Design review of the part built by this model. Coordinates are the model's own, in mm. Face numbers are marked on the shaded views. A direction names the side the tool comes from. Round coordinates to 2 decimals unless told otherwise and drop trailing zeros. Write each loop counter-clockwise with the first axis right and the second up, starting at its lowest first coordinate (ties: lowest second). Pieces come first, ordered by that corner, then holes. Notation, with made-up numbers: M -16.75,23.25 L 3.25,23.25 A22 cw 3.25,47.25 Z; hole C 79.5,16 d5. An arc over 180 degrees is marked long. Use CSV: the item, a comma, the result in double quotes.
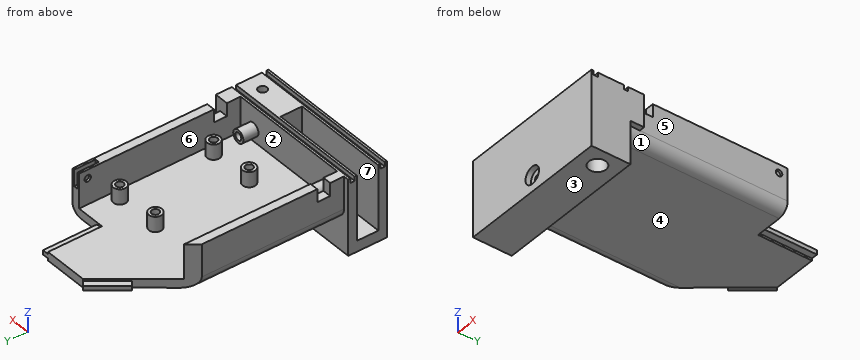
from build123d import *

# Parameters (mm, degrees)
SKETCH1_W                 = 65
SKETCH1_H                 = 40
BOSS_EXTRUDE1_DEPTH       = 100
SHELL1_T                  = -4
FILLET1_R                 = 5
CUT_EXTRUDE1_DEPTH        = 108.033873143
CUT_EXTRUDE1_DEPTH_BACK   = 108.033873143
CUT_EXTRUDE2_DEPTH        = 108.033873143
CUT_EXTRUDE2_DEPTH_BACK   = 108.033873143
SKETCH3_W                 = 17.5
SKETCH3_H                 = 25
SKETCH5_W                 = 2
SKETCH5_H                 = 25
BOSS_EXTRUDE2_DEPTH       = 3
SKETCH6_W                 = 2
SKETCH6_H                 = 18
BOSS_EXTRUDE3_DEPTH       = 3
SKETCH8_W                 = 70
SKETCH8_H                 = 70
BOSS_EXTRUDE4_DEPTH       = 18
SKETCH10_W                = 60
SKETCH10_H                = 10
CUT_EXTRUDE4_DEPTH        = 45
SKETCH23_W                = 2
SKETCH23_H                = 15
CUT_EXTRUDE10_DEPTH       = 10
CUT_EXTRUDE12_DEPTH       = 114.254624289
CUT_EXTRUDE12_DEPTH_BACK  = 114.254624289
SKETCH27_W                = 70
SKETCH27_H                = 35
SKETCH29_W                = 70
SKETCH29_H                = 2
CUT_EXTRUDE13_DEPTH       = 2
SKETCH30_W                = 70
SKETCH30_H                = 2
CUT_EXTRUDE14_DEPTH       = 2
CUT_EXTRUDE15_DEPTH       = 114.254624289
CUT_EXTRUDE15_DEPTH_BACK  = 114.254624289
SKETCH31_R                = 2
SKETCH33_R                = 4
CUT_EXTRUDE16_DEPTH       = 15
CUT_EXTRUDE17_DEPTH       = 114.254624289
CUT_EXTRUDE17_DEPTH_BACK  = 114.254624289
SKETCH34_R                = 1.5
SKETCH35_R                = 4
CUT_EXTRUDE18_DEPTH       = 2.5
SKETCH39_R                = 3
BOSS_EXTRUDE7_DEPTH       = 7
SKETCH40_R                = 1.75
CUT_EXTRUDE20_DEPTH       = 4
LPATTERN4_COUNT           = 2
LPATTERN4_PITCH           = 43.5
CUT_EXTRUDE21_DEPTH       = 128.113570962
CUT_EXTRUDE21_DEPTH_BACK  = 128.113570962
SKETCH41_W                = 6
SKETCH41_H                = 6
SKETCH42_W                = 15
SKETCH42_H                = 6.4
BOSS_EXTRUDE10_DEPTH      = 2.5
CUT_EXTRUDE22_DEPTH       = 128.113570962
CUT_EXTRUDE22_DEPTH_BACK  = 10
SKETCH43_R                = 1.5
SKETCH37_R                = 3
BOSS_EXTRUDE6_DEPTH       = 7
SKETCH38_R                = 1.75
CUT_EXTRUDE19_DEPTH       = 4
LPATTERN1_COUNT           = 2
LPATTERN1_PITCH           = 21
LPATTERN2_COUNT           = 2
LPATTERN2_PITCH           = 43.5
LPATTERN2_COPY_1_SKETCH_R = 3
LPATTERN2_COPY_1_DEPTH    = 7
LPATTERN2_COPY_2_SKETCH_R = 1.75
LPATTERN2_COPY_2_DEPTH    = 4


with BuildPart() as part:
    # Sketch1 → Boss-Extrude1 (new body)
    with BuildSketch(Plane(origin=(0, 0, 0), x_dir=(1, 0, 0), z_dir=(0, 1, 0))):
        Rectangle(SKETCH1_W, SKETCH1_H)
    extrude(amount=BOSS_EXTRUDE1_DEPTH)

    # Shell1
    shell1_openings = [part.faces().sort_by_distance(p)[0] for p in [
        (0, 100, 0),
        (0, 0, 0),
    ]]
    offset(amount=SHELL1_T, openings=shell1_openings, kind=Kind.INTERSECTION)

    # Fillet1
    fillet1_edges = [part.edges().sort_by_distance(p)[0] for p in [
        (32.5, 50, 20),
        (-32.5, 50, 20),
        (-32.5, 50, -20),
        (32.5, 50, -20),
    ]]
    fillet(fillet1_edges, radius=FILLET1_R)

    # Sketch2 → Cut-Extrude1 (cut, two sides: drawn at the far end of the back side and taken through both)
    with BuildSketch(Plane.XY.offset(-CUT_EXTRUDE1_DEPTH_BACK)):
        Polygon((-5.5, 100), (-32.5, 66), (-32.5, 100), align=None)
    extrude(amount=CUT_EXTRUDE1_DEPTH + CUT_EXTRUDE1_DEPTH_BACK, mode=Mode.SUBTRACT)

    # Sketch3 → Cut-Extrude2 (cut, two sides: drawn at the far end of the back side and taken through both)
    with BuildSketch(Plane.XY.offset(-CUT_EXTRUDE2_DEPTH_BACK)):
        with Locations((23.75, 87.5)):
            Rectangle(SKETCH3_W, SKETCH3_H)
    extrude(amount=CUT_EXTRUDE2_DEPTH + CUT_EXTRUDE2_DEPTH_BACK, mode=Mode.SUBTRACT)

    # Sketch5 → Boss-Extrude2 (add)
    with BuildSketch(Plane(origin=(15, 0, 0), x_dir=(0, 0, -1), z_dir=(1, 0, 0))):
        with Locations((-18, 87.5)):
            Rectangle(SKETCH5_W, SKETCH5_H)
    boss_extrude2 = extrude(amount=BOSS_EXTRUDE2_DEPTH)

    # Mirror1: Boss-Extrude2 across plane
    add(boss_extrude2.mirror(Plane.XY))

    # Sketch6 → Boss-Extrude3 (add)
    with BuildSketch(Plane(origin=(-52.073209549, 41.352254642, 0), x_dir=(0, 0, 1), z_dir=(-0.783110847498294, 0.6218821436015861, 0))):
        with Locations((-18, 65.89073296)):
            Rectangle(SKETCH6_W, SKETCH6_H)
    boss_extrude3 = extrude(amount=BOSS_EXTRUDE3_DEPTH)

    # Mirror2: Boss-Extrude3 across plane
    add(boss_extrude3.mirror(Plane.XY))

    # Sketch8 → Boss-Extrude4 (add)
    with BuildSketch(Plane(origin=(0, 0, 0), x_dir=(1, 0, 0), z_dir=(0, 1, 0))):
        Rectangle(SKETCH8_W, SKETCH8_H)
    extrude(amount=-BOSS_EXTRUDE4_DEPTH)

    # Sketch10 → Cut-Extrude4 (cut)
    with BuildSketch(Plane.ZY.offset(35)):
        with Locations((0, -9)):
            Rectangle(SKETCH10_W, SKETCH10_H)
    extrude(amount=-CUT_EXTRUDE4_DEPTH, mode=Mode.SUBTRACT)

    # Sketch23 → Cut-Extrude10 (cut)
    with BuildSketch(Plane(origin=(0, 75, 0), x_dir=(1, 0, 0), z_dir=(0, 1, 0))):
        with Locations((30.5, 0)):
            Rectangle(SKETCH23_W, SKETCH23_H)
    extrude(amount=-CUT_EXTRUDE10_DEPTH, mode=Mode.SUBTRACT)

    # Sketch27 → Cut-Extrude12 (cut, two sides: drawn at the far end of the back side and taken through both)
    with BuildSketch(Plane(origin=(0, 0, 0), x_dir=(1, 0, 0), z_dir=(0, 1, 0)).offset(-CUT_EXTRUDE12_DEPTH_BACK)):
        with Locations((0, -17.5)):
            Rectangle(SKETCH27_W, SKETCH27_H)
    extrude(amount=CUT_EXTRUDE12_DEPTH + CUT_EXTRUDE12_DEPTH_BACK, mode=Mode.SUBTRACT)

    # Sketch29 → Cut-Extrude13 (cut)
    with BuildSketch(Plane.XY):
        with Locations((0, -2)):
            Rectangle(SKETCH29_W, SKETCH29_H)
    extrude(amount=-CUT_EXTRUDE13_DEPTH, mode=Mode.SUBTRACT)

    # Sketch30 → Cut-Extrude14 (cut)
    with BuildSketch(Plane.XY):
        with Locations((0, -16)):
            Rectangle(SKETCH30_W, SKETCH30_H)
    extrude(amount=-CUT_EXTRUDE14_DEPTH, mode=Mode.SUBTRACT)

    # Sketch31 → Cut-Extrude15 (cut, two sides: drawn at the far end of the back side and taken through both)
    with BuildSketch(Plane.XY.offset(-CUT_EXTRUDE15_DEPTH_BACK)):
        with Locations((27, -9)):
            Circle(SKETCH31_R)
    extrude(amount=CUT_EXTRUDE15_DEPTH + CUT_EXTRUDE15_DEPTH_BACK, mode=Mode.SUBTRACT)

    # Sketch33 → Cut-Extrude16 (cut)
    with BuildSketch(Plane(origin=(0, 0, -35), x_dir=(-1, 0, 0), z_dir=(0, 0, -1))):
        with Locations((-27, -9)):
            Circle(SKETCH33_R)
    extrude(amount=-CUT_EXTRUDE16_DEPTH, mode=Mode.SUBTRACT)

    # Sketch34 → Cut-Extrude17 (cut, two sides: drawn at the far end of the back side and taken through both)
    with BuildSketch(Plane(origin=(0, 0, 0), x_dir=(1, 0, 0), z_dir=(0, 1, 0)).offset(-CUT_EXTRUDE17_DEPTH_BACK)):
        with Locations(Location((0, 27.5, 0), (0, 0, 270))):
            Circle(SKETCH34_R)
    extrude(amount=CUT_EXTRUDE17_DEPTH + CUT_EXTRUDE17_DEPTH_BACK, mode=Mode.SUBTRACT)

    # Sketch35 → Cut-Extrude18 (cut)
    with BuildSketch(Plane(origin=(0, -18, 0), x_dir=(-1, 0, 0), z_dir=(0, -1, 0))):
        with Locations(Location((0, 27.5, 0), (0, 0, 90))):
            Circle(SKETCH35_R)
    extrude(amount=-CUT_EXTRUDE18_DEPTH, mode=Mode.SUBTRACT)

    # Sketch39 → Boss-Extrude7 (add)
    with BuildSketch(Plane(origin=(0, 0, 0), x_dir=(1, 0, 0), z_dir=(0, 1, 0))):
        with Locations(Location((21, 10.5, 0), (0, 0, 90))):
            Circle(SKETCH39_R)
    boss_extrude7 = extrude(amount=BOSS_EXTRUDE7_DEPTH)

    # Sketch40 → Cut-Extrude20 (cut)
    with BuildSketch(Plane(origin=(0, 7, 0), x_dir=(1, 0, 0), z_dir=(0, 1, 0))):
        with Locations(Location((21, 10.5, 0), (0, 0, 270))):
            Circle(SKETCH40_R)
    cut_extrude20 = extrude(amount=-CUT_EXTRUDE20_DEPTH, mode=Mode.SUBTRACT)

    # LPattern4: Boss-Extrude7, Cut-Extrude20 ×2
    with Locations(*[(-i * LPATTERN4_PITCH, 0, 0) for i in range(1, LPATTERN4_COUNT)]):
        add(boss_extrude7)
        add(cut_extrude20, mode=Mode.SUBTRACT)

    # Sketch41 → Cut-Extrude21 (cut, two sides: drawn at the far end of the back side and taken through both)
    with BuildSketch(Plane(origin=(32.5, 0, 0), x_dir=(0, 0, -1), z_dir=(1, 0, 0)).offset(-CUT_EXTRUDE21_DEPTH_BACK)):
        with Locations((3, 9.4)):
            Rectangle(SKETCH41_W, SKETCH41_H)
    extrude(amount=CUT_EXTRUDE21_DEPTH + CUT_EXTRUDE21_DEPTH_BACK, mode=Mode.SUBTRACT)

    # Sketch42 → Boss-Extrude10 (add)
    with BuildSketch(Plane(origin=(32.5, 0, 0), x_dir=(0, 0, -1), z_dir=(1, 0, 0))):
        with Locations((7.5, 3.2)):
            Rectangle(SKETCH42_W, SKETCH42_H)
    extrude(amount=BOSS_EXTRUDE10_DEPTH)

    # Sketch43 → Cut-Extrude22 (cut, two sides: drawn at the far end of the back side and taken through both)
    with BuildSketch(Plane(origin=(32.5, 0, 0), x_dir=(0, 0, -1), z_dir=(1, 0, 0)).offset(-CUT_EXTRUDE22_DEPTH_BACK)):
        with Locations(Location((4, 71, 0), (0, 0, 180))):
            Circle(SKETCH43_R)
    extrude(amount=CUT_EXTRUDE22_DEPTH + CUT_EXTRUDE22_DEPTH_BACK, mode=Mode.SUBTRACT)

    # Sketch37 → Boss-Extrude6 (add)
    with BuildSketch(Plane.XY.offset(-16)):
        with Locations(Location((23.5, 60, 0), (0, 0, 180))):
            Circle(SKETCH37_R)
    boss_extrude6 = extrude(amount=BOSS_EXTRUDE6_DEPTH)

    # Sketch38 → Cut-Extrude19 (cut)
    with BuildSketch(Plane.XY.offset(-9)):
        with Locations((23.5, 60)):
            Circle(SKETCH38_R)
    cut_extrude19 = extrude(amount=-CUT_EXTRUDE19_DEPTH, mode=Mode.SUBTRACT)

    # LPattern1: Boss-Extrude6, Cut-Extrude19 ×2
    with Locations(*[(-i * LPATTERN1_PITCH, 0, 0) for i in range(1, LPATTERN1_COUNT)]):
        add(boss_extrude6)
        add(cut_extrude19, mode=Mode.SUBTRACT)

    # LPattern2: Boss-Extrude6, Cut-Extrude19 ×2
    with Locations(*[(0, -i * LPATTERN2_PITCH, 0) for i in range(1, LPATTERN2_COUNT)]):
        add(boss_extrude6)
        add(cut_extrude19, mode=Mode.SUBTRACT)

    # LPattern2 copy 1 sketch → LPattern2 copy 1 (add)
    with BuildSketch(Plane(origin=(-21, -43.5, -16), x_dir=(1, 0, 0), z_dir=(0, 0, 1))):
        with Locations(Location((23.5, 60, 0), (0, 0, 180))):
            Circle(LPATTERN2_COPY_1_SKETCH_R)
    extrude(amount=LPATTERN2_COPY_1_DEPTH)

    # LPattern2 copy 2 sketch → LPattern2 copy 2 (cut)
    with BuildSketch(Plane(origin=(-21, -43.5, -9), x_dir=(1, 0, 0), z_dir=(0, 0, 1))):
        with Locations((23.5, 60)):
            Circle(LPATTERN2_COPY_2_SKETCH_R)
    extrude(amount=-LPATTERN2_COPY_2_DEPTH, mode=Mode.SUBTRACT)


solid = part.part
1) Machinability: for the marked faces 4, 5, 6 and 7, which of the approach directions +Z, -Z, +X, -X, +Y, -Y give a long, thin tool a straight path to every point of the face, cutting with its end or side? Answer none if there is none.
Answers:
face 4,"-Z, +X, -X, +Y"
face 5,"+Z, -Z, +X, +Y"
face 6,"+Z, +Y"
face 7,"+Z, -X"
2) Add section A-A on z = -27.5. Write out the cut boundary in (x, y), then the cut area to 3 significant figures.
Answers:
outline,"M -35,-18 L -4,-18 L -4,-15.5 L -1.5,-15.5 L -1.5,-14 L -35,-14 Z; M -35,-4 L -1.5,-4 L -1.5,0 L -35,0 Z; M 1.5,-15.5 L 4,-15.5 L 4,-18 L 35,-18 L 35,0 L 1.5,0 L 1.5,-4 L 10,-4 L 10,-14 L 1.5,-14 Z; hole C 27,-9 d8"
area,"723 mm²"
3) Add section D-D on z = -10.5. Give the number of separate pieces and of enclosed holes in the cut face, then the cut area to 3 significant figures.
Answers:
separate pieces,"5"
enclosed holes,"5"
area,"1,520 mm²"
4) Add section B-B on y = -9. Write out the cut boundary in (x, z).
Answers:
outline,"M -35,-35 L 23,-35 L 23,-20 L 25,-20 L 25,0 L 10,0 L 10,-30 L -35,-30 Z; M 29,-20 L 31,-20 L 31,-35 L 35,-35 L 35,0 L 29,0 Z"
5) Add section C-C on y = 43.5. Write out the cut boundary in (x, z), then the cut area to 3 significant figures.
Answers:
outline,"M -32.5,-15 A5 ccw -27.5,-20 L 27.5,-20 A5 ccw 32.5,-15 L 32.5,0 L 28.5,0 L 28.5,-16 L -28.5,-16 L -28.5,0 L -32.5,0 Z"
area,"377 mm²"
6) Wall thickness on line 1 along Y through (x, z) = (-6, -1.5); line 2 along Y through (x, z) = (-16.5, -23.5); line 3 along Y through (x, z) = (-24.5, -10): over which ranges is each line inside the solid? List them lowest first. Write a range as [from, to].
Answers:
line 1,"[-18, -17], [-15, -14], [-4, -3], [-1, 0]"
line 2,"[-18, -14], [-4, 0]"
line 3,"[-18, -14], [-4, 7]"
7) The part is to be moulded in two halves that separate along X. For the marked faces 1, 2 and 3, say which applies: released by +X, released by -X, zero draft, split by the parting line, or undercut.
Answers:
face 1,"released by +X"
face 2,"undercut"
face 3,"zero draft"
8) For pin 1 Ø1 at (x, y) = (2.5, 60) entering from +Z; pin 2 Ø3.5 at (x, z) = (0, -27.5) entering from +Y; pin 3 Ø7 at (x, y) = (-14.5, 94) entering from +Z; pin 4 Ø10 at (x, z) = (-7.5, -23.5) entering from +Y, all flat-tipped, find the tip position at first contact; note any pin that passes through.
Answers:
pin 1,"z = -13"
pin 2,"y = 0"
pin 3,"z = -16"
pin 4,"y = 101.87"
